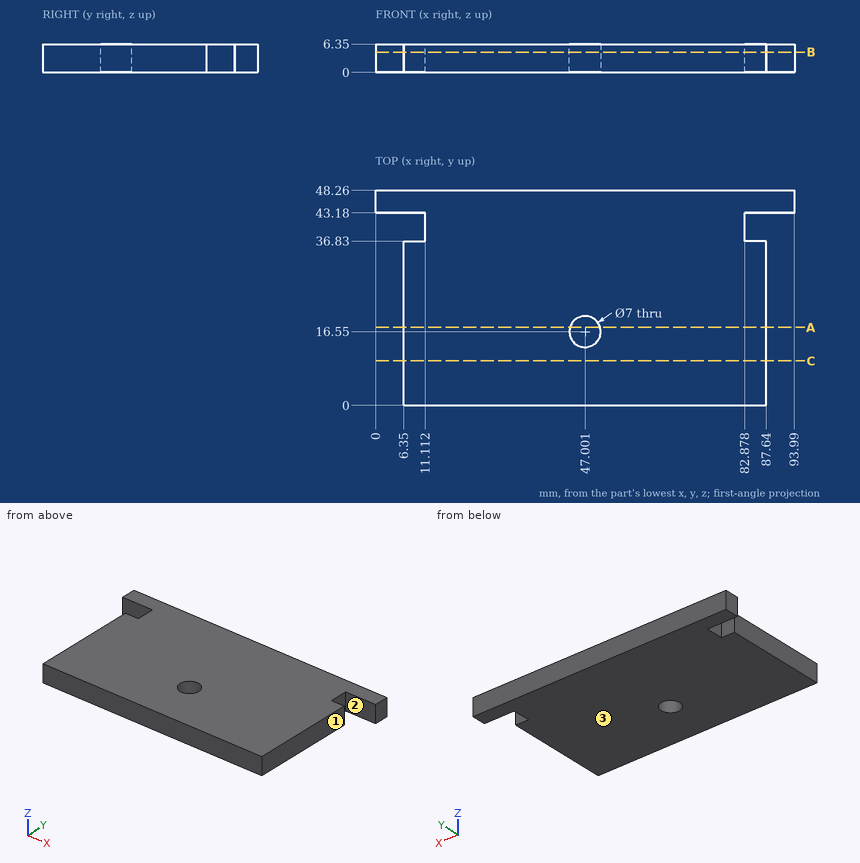
The drawing under review shows one solid part. Ordinate dimensions are in mm from its lowest x, y, z. A direction names the side the tool comes from. Round coordinates to 2 decimals unless told otherwise and drop trailing zeros. Write each loop counter-clockwise with the first axis right and the second up, starting at its lowest first coordinate (ties: lowest second). Pieces come first, ordered by that corner, then holes. Notation, with made-up numbers: (-16, 2) -> (36, 2) arc R22 ccw to (36, 19) -> close; hole circle Ø4 at (89, 57.25). An arc over 180 degrees is marked (long way). One line per question, with ' | ' between items.
(1) Take a section at A-A, the plane y = 17.5. State the section outline as (x, z) points.
Result sheet:
outline: (6.35, 0) -> (43.63, 0) -> (43.63, 6.35) -> (6.35, 6.35) -> close; (50.37, 0) -> (87.64, 0) -> (87.64, 6.35) -> (50.37, 6.35) -> close
(2) Take a section at B-B, the plane z = 4.5. State the section outline as (x, y) points.
Result sheet:
outline: (0, 43.18) -> (11.11, 43.18) -> (11.11, 36.83) -> (6.35, 36.83) -> (6.35, 0) -> (87.64, 0) -> (87.64, 36.83) -> (82.88, 36.83) -> (82.88, 43.18) -> (93.99, 43.18) -> (93.99, 48.26) -> (0, 48.26) -> close; hole circle Ø7 at (47, 16.55)
(3) Wall thickness on line 1 (Y direction, x = 10, z = 4.5); line 2 (X direction, y = 24.5, z = 0.5); line 3 (Y direction, x = 6, z = 5.75): over which ranges is each line inside the solid? List them lowest first. Write a range as [from, to].
Result sheet:
line 1: [0, 36.83], [43.18, 48.26] | line 2: [6.35, 87.64] | line 3: [43.18, 48.26]
(4) Insertion check: P1, Ø3, axis at y = 40.5, z = 2.5, coming from the -X side; P2, Ø1, axis at y = 13.5, z = 1.5, coming from the -X side; P3, Ø3, axis at y = 18, z = 4, coming from the +X side; P4, Ø6.5, axis at x = 47, y = 16.55, coming from the +Z side. Each pin has a flat end and moves straight along its axis. Give the tip position at first contact, or say it passes through.
Result sheet:
P1: x = 11.11 | P2: x = 6.35 | P3: x = 87.64 | P4: through
(5) Take a section at C-C, the plane y = 10. State the section outline as (x, z) points, and give its area (3 significant figures).
Result sheet:
outline: (6.35, 0) -> (87.64, 0) -> (87.64, 6.35) -> (6.35, 6.35) -> close | area: 516 mm2
(6) Machinability: for the marked faces 1, 2 and 3, which of the approach directions +Z, -Z, +X, -X, +Y, -Y give a long, thin tool a straight path to every point of the face, cutting with its end or side? Answer none if there is none.
Result sheet:
face 1: +Z, -Z, +X, -Y | face 2: +Z, -Z, +X | face 3: -Z, +X, -X, +Y, -Y
